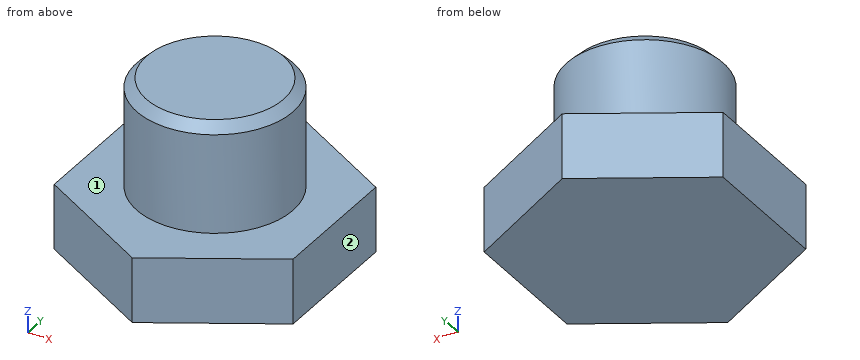
from build123d import *

# Parameters (mm, degrees)
EXTRUDE_1_DEPTH = 15
SKETCH_2_R      = 18
EXTRUDE_2_DEPTH = 25
CHAMFER_1_SIZE  = 2.195


with BuildPart() as part:
    # Эскиз1 → Бобышка-Вытянуть1 (new body)
    with BuildSketch(Plane.XY):
        Polygon((0, 31.754264805), (-27.5, 15.877132403), (-27.5, -15.877132403), (0, -31.754264805), (27.5, -15.877132403), (27.5, 15.877132403), align=None)
    extrude(amount=EXTRUDE_1_DEPTH)

    # Эскиз2 → Бобышка-Вытянуть2 (add)
    with BuildSketch(Plane.XY.offset(15)):
        Circle(SKETCH_2_R)
    extrude(amount=EXTRUDE_2_DEPTH)

    # Фаска1
    chamfer_1_edges = [part.edges().sort_by_distance(p)[0] for p in [
        (-18, 0, 40),
    ]]
    chamfer(chamfer_1_edges, length=CHAMFER_1_SIZE)


solid = part.part
Input: part model. Units: mm. Frame: model coordinates. Face numbers are marked on the shaded views. A direction names the side the tool comes from. Give positions to 0.01 mm unless a question says otherwise; leave off trailing zeros. Write each loop counter-clockwise with the first axis right and the second up, starting at its lowest first coordinate (ties: lowest second). Pieces come first, ordered by that corner, then holes. Notation, with made-up numbers: (83.5, 38) -> (137.5, 38) arc R17 ccw to (137.5, 51) -> close; hole circle Ø10 at (39, -37.75). An arc over 180 degrees is marked (long way). Use one line per item in the form item = value. Start each with the question number.
1) Pin query (flat end, axial travel): pin 1 (5 mm diameter, centred on x = -20.5, z = 15.5, fed in from -Y); pin 2 (4 mm diameter, centred on x = -14, y = -18.5, fed in from +Z); pin 3 (3 mm diameter, centred on x = 10, y = -16, fed in from +Z). Return the tip coordinate at first contact, or that it passes through.
2) Section query C-C on x = -20.5. Return the cut outline in (y, z), then the cut area to 3 significant figures.
3) Section query D-D on z = 31. Return the cut outline in (x, y), then the cut area to 3 significant figures.
4) Set-up query: the marked faces 1 and 2. Return all of +Z, -Z, +X, -X, +Y, -Y with unobstructed straight access to the full face (end or side cutting, diameter ignored); none if empty.
5) Section query B-B on y = 0. Return the cut outline in (x, z) (3 decimals).
6) Section query A-A on z = 6.5. Return the cut outline in (x, y), then the cut area to 3 significant figures.
7) Ray query, probe 1 along Z at (x, y) = (-19, 0.5); probe 2 along X at (y, z) = (21, 14); probe 3 along Y at (x, z) = (3, 13.5). Return the intervals inside material, ascending. Write a range as from..to.
Outcome:
q1.pin_1 = -21.33
q1.pin_2 = 15
q1.pin_3 = 38.44
q2.outline = (-19.92, 0) -> (19.92, 0) -> (19.92, 15) -> (-19.92, 15) -> close
q2.area = 598 mm^2
q3.outline = circle Ø36 at (0, 0)
q3.area = 1,020 mm^2
q4.face_1 = +Z
q4.face_2 = +Z, -Z, +X, +Y, -Y
q5.outline = (-27.5, 0) -> (27.5, 0) -> (27.5, 15) -> (18, 15) -> (18, 37.805) -> (15.805, 40) -> (-15.805, 40) -> (-18, 37.805) -> (-18, 15) -> (-27.5, 15) -> close
q6.outline = (-27.5, -15.88) -> (0, -31.75) -> (27.5, -15.88) -> (27.5, 15.88) -> (0, 31.75) -> (-27.5, 15.88) -> close
q6.area = 2,620 mm^2
q7.probe_1 = 0..15
q7.probe_2 = -18.63..18.63
q7.probe_3 = -30.02..30.02
